Could you check a few things on this model? Use its own coordinates, in mm. Give positions to 0.01 mm unless a question says otherwise; leave off trailing zeros. Order: outer loops, then holes, each group sorted by start corner. A loop starts at its lowest first (then second) coordinate and runs counter-clockwise, first axis right, second up.
(1) Imagine slicing it at B-B, the plane x = 15.5. Write out the boundary of the cut face in (y, z) (1 decimal).
(2) Will this pin go through, and if not, where does the flat tip stop? pin 1 (2 mm diameter, centred on x = 41, z = -31.83, fed in from -Y).
(3) If I drill on probe 1 along X at (y, z) = (-2.2, -18.5); probe 2 along Z at (x, y) = (-14, 1.55) (1 decimal); probe 3 along Z at (x, y) = (44.5, 2.15) (1 decimal), over which ranges is the centre line in solid material (lowest first)?
(4) Imagine slicing it at C-C, the plane y = -1.3. State how many separate pieces and enclosed holes the cut face has, then the cut area to 3 significant figures.
(5) Imagine slicing it at A-A, the plane z = 23. Write out the boundary of the cut face in (x, y), then the cut area to 3 significant figures.
(6) If we mould it in two halves opening along Z, with no side actions, what happens to faces 1 (the flat face through (-54.229, 0, 1)), 2 (the flat face through (48.92, 0, -23)), 3 (the cylindrical face through (-52.96, -0.04, -50.1))? For each: released by +Z, released by -Z, zero draft, split by the parting line, or undercut.
from build123d import *

# Parameters (mm, degrees)
SKETCH1_W           = 108.458
SKETCH1_H           = 102.87
SKETCH1_R           = 1.1303
SKETCH1_W_2         = 3.2766
SKETCH1_H_2         = 32.1564
BOSS_EXTRUDE1_DEPTH = 2.7178
FILLET1_R           = 4.445
SKETCH3_W           = 5.334
SKETCH3_H           = 4.953
CUT_EXTRUDE2_DEPTH  = 75.939238142


with BuildPart() as part:
    # Sketch1 → Boss-Extrude1 (new, symmetric)
    with BuildSketch(Plane(origin=(0, 0, 0), x_dir=(1, 0, 0), z_dir=(0, 1, 0))):
        Rectangle(SKETCH1_W, SKETCH1_H)
        with Locations(Location((-40.9956, -29.1846, 0), (0, 0, 270))):
            Circle(SKETCH1_R, mode=Mode.SUBTRACT)
        with Locations(Location((40.9956, -29.1846, 0), (0, 0, 90))):
            Circle(SKETCH1_R, mode=Mode.SUBTRACT)
        with Locations(Location((-40.9956, 31.8262, 0), (0, 0, 270))):
            Circle(SKETCH1_R, mode=Mode.SUBTRACT)
        with Locations(Location((40.9956, 31.8262, 0), (0, 0, 90))):
            Circle(SKETCH1_R, mode=Mode.SUBTRACT)
        Polygon((41.7322, 46.126399066), (41.7322, 49.403), (9.548058937, 49.403), (9.578119675, 46.126517444), align=None, mode=Mode.SUBTRACT)
        Polygon((-9.578119675, 46.126517444), (-9.548058937, 49.403), (-41.7322, 49.403), (-41.7322, 46.126399066), align=None, mode=Mode.SUBTRACT)
        with Locations((50.5587, -22.86)):
            Rectangle(SKETCH1_W_2, SKETCH1_H_2, mode=Mode.SUBTRACT)
        with Locations((50.5587, 22.86)):
            Rectangle(SKETCH1_W_2, SKETCH1_H_2, mode=Mode.SUBTRACT)
        Polygon((41.7322, -46.126399065), (9.578119675, -46.126517443), (9.548058937, -49.403), (41.7322, -49.403), align=None, mode=Mode.SUBTRACT)
        Polygon((-41.7322, -46.126399065), (-41.7322, -49.403), (-9.548058937, -49.403), (-9.578119675, -46.126517443), align=None, mode=Mode.SUBTRACT)
        with Locations((-50.5587, 22.86)):
            Rectangle(SKETCH1_W_2, SKETCH1_H_2, mode=Mode.SUBTRACT)
        with Locations((-50.5587, -22.86)):
            Rectangle(SKETCH1_W_2, SKETCH1_H_2, mode=Mode.SUBTRACT)
    extrude(amount=BOSS_EXTRUDE1_DEPTH, both=True)

    # Fillet1
    fillet1_edges = [part.edges().sort_by_distance(p)[0] for p in [
        (-54.229, 0, -51.435),
        (54.229, 0, -51.435),
        (54.229, 0, 51.435),
        (-54.229, 0, 51.435),
    ]]
    fillet(fillet1_edges, radius=FILLET1_R)

    # Sketch3 → Cut-Extrude2 (cut, through all)
    with BuildSketch(Plane(origin=(0, 2.7178, 0), x_dir=(1, 0, 0), z_dir=(0, 1, 0))):
        with Locations((44.323, -38.735)):
            Rectangle(SKETCH3_W, SKETCH3_H)
    extrude(amount=-CUT_EXTRUDE2_DEPTH, mode=Mode.SUBTRACT)


solid = part.part
Answer block:
1. outline: (-2.7, -51.4) - (2.7, -51.4) - (2.7, -49.4) - (-2.7, -49.4) - close; (-2.7, -46.1) - (2.7, -46.1) - (2.7, 46.1) - (-2.7, 46.1) - close; (-2.7, 49.4) - (2.7, 49.4) - (2.7, 51.4) - (-2.7, 51.4) - close
2. pin 1: passes through
3. probe 1: x = -54.23 to -52.2, -48.92 to 48.92, 52.2 to 54.23
3. probe 2: z = -51.4 to -49.4, -46.1 to 46.1, 49.4 to 51.4
3. probe 3: z = -51.4 to 36.3, 41.2 to 51.4
4. separate pieces: 1
4. enclosed holes: 13
4. area: 10,300 mm2
5. outline: (-54.23, -2.72) - (-52.2, -2.72) - (-52.2, 2.72) - (-54.23, 2.72) - close; (-48.92, -2.72) - (48.92, -2.72) - (48.92, 2.72) - (-48.92, 2.72) - close; (52.2, -2.72) - (54.23, -2.72) - (54.23, 2.72) - (52.2, 2.72) - close
5. area: 554 mm2
6. face 1: zero draft
6. face 2: undercut
6. face 3: released by -Z
